The listing builds one solid part. Answer for the finished solid, in the listing's coordinates (mm). Face numbers are marked on the shaded views. A direction names the side the tool comes from. Give positions to 0.01 mm unless a question says otherwise; leave off trailing zeros. Write each loop counter-clockwise with the first axis right and the second up, starting at its lowest first coordinate (ties: lowest second). Pieces come first, ordered by that corner, then holes. Notation, with made-up numbers: M -11.75,83 L 31.25,83 A19 ccw 31.25,109 Z; hole C 8.25,-11.75 d5. An arc over 180 degrees is marked long. Return JSON: item names as keys, results as strings.
from build123d import *

# Parameters (mm, degrees)
F0_W     = 1.524
F0_H     = 2.54
F1_DEPTH = 6.35
F2_R     = 0.508


with BuildPart() as f1:
    # F0 (on Top) → F1 (new body)
    with BuildSketch(Plane.XY):
        Polygon((3.81, 4.064), (5.334, 4.064), (5.334, 5.588), (0, 5.588), (0, 4.064), align=None)
        with Locations((4.572, 2.794)):
            Rectangle(F0_W, F0_H)
        Polygon((0, 1.524), (0, 0), (5.334, 0), (5.334, 1.524), (3.81, 1.524), align=None)
    extrude(amount=F1_DEPTH)

    # F2
    f2_edges = [f1.edges().sort_by_distance(p)[0] for p in [
        (0, 4.064, 3.175),
        (0, 5.588, 3.175),
        (0, 1.524, 3.175),
        (0, 0, 3.175),
        (5.334, 0, 3.175),
        (5.334, 5.588, 3.175),
    ]]
    fillet(f2_edges, radius=F2_R)


solid = f1.part
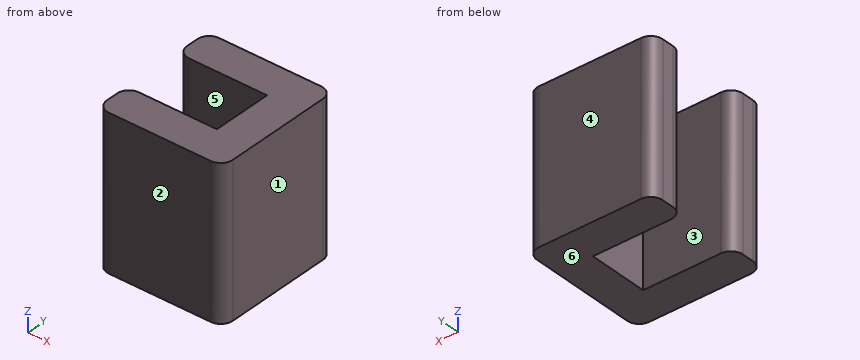
Item 1: Which of the six approach directions +Z, -Z, +X, -X, +Y, -Y give full straight-line access (tool end or side, diameter ignored) to the marked faces 5 and 6?
Geometry results:
{"face 5": "+Z, -Z, -X", "face 6": "-Z, +X, -X, +Y, -Y"}
Item 2: A cutting plane is placed at D-D, the plane x = 0.35. Write down the section's boundary in (y, z).
Geometry results:
{"outline": "M 0.03,0 L 1.5,0 L 1.5,6.35 L 0.03,6.35 Z; M 4.09,0 L 5.56,0 L 5.56,6.35 L 4.09,6.35 Z"}
Item 3: A cutting plane is placed at C-C, the plane y = 1.75. Write down the section's boundary in (x, z), plus the area to 3 significant figures.
Geometry results:
{"outline": "M 3.81,0 L 5.33,0 L 5.33,6.35 L 3.81,6.35 Z", "area": "9.68 mm2"}
Item 4: A cutting plane is placed at B-B, the plane z = 3.5. Write down the section's boundary in (x, y).
Geometry results:
{"outline": "M 0,0.51 A0.51 ccw 0.51,0 L 4.83,0 A0.51 ccw 5.33,0.51 L 5.33,5.08 A0.51 ccw 4.83,5.59 L 0.51,5.59 A0.51 ccw 0,5.08 L 0,4.57 A0.51 ccw 0.51,4.06 L 3.81,4.06 L 3.81,1.52 L 0.51,1.52 A0.51 ccw 0,1.02 Z"}
Item 5: A cutting plane is placed at A-A, the plane x = 3.7. Write down the section's boundary in (y, z), plus the area to 3 significant figures.
Geometry results:
{"outline": "M 0,0 L 1.52,0 L 1.52,6.35 L 0,6.35 Z; M 4.06,0 L 5.59,0 L 5.59,6.35 L 4.06,6.35 Z", "area": "19.4 mm2"}
Item 6: Determine the mould class of the marked faces 1, 2, 3 and 4 for opening direction Y: +Y half, -Y half, draft (parallel to the pull), parting line (faces both ways), or undercut.
Geometry results:
{"face 1": "draft", "face 2": "-Y half", "face 3": "undercut", "face 4": "+Y half"}
Item 7: Find the intervals of material crossed by line 1 (Y direction, x = 3.3, z = 0.5); line 2 (X direction, y = 2.4, z = 2.75); line 3 (X direction, y = 4.25, z = 6), in increasing order.
Geometry results:
{"line 1": "y = 0 to 1.52, 4.06 to 5.59", "line 2": "x = 3.81 to 5.33", "line 3": "x = 0.12 to 5.33"}
Item 8: Given pin 1 Ø1.5 at (y, z) = (2, 1) entering from -X; pin 2 Ø1.3 at (y, z) = (2.5, 4) entering from -X, each flat-ended and moving along its own axis, determine where each tip first touches the part or whether it passes through.
Geometry results:
{"pin 1": "stops at x = 0.06", "pin 2": "stops at x = 3.81"}
